Read the model definition and answer for the solid it produces. Units are mm, in the model's axes. Give positions to 0.01 mm unless a question says otherwise; leave off trailing zeros. Write each loop counter-clockwise with the first axis right and the second up, starting at its lowest first coordinate (ties: lowest second). Pieces come first, ordered by that corner, then holes. Notation, with made-up numbers: (7, 81) - (41, 81) arc R27 cw to (41, 108) - close; hole circle Ø6 at (1.5, -22). An arc over 180 degrees is marked (long way). Answer as a JSON object with one key per item and string values. Group by question number.
```python
from build123d import *

# Parameters (mm, degrees)
SKETCH1_R           = 17.5
BOSS_EXTRUDE1_DEPTH = 1.5
SKETCH2_R           = 7
SKETCH2_R_2         = 1.5
CUT_EXTRUDE1_DEPTH  = 1.5
CHAMFER1_SIZE       = 0.75
CHAMFER2_SIZE       = 0.25


with BuildPart() as part:
    # Sketch1 → Boss-Extrude1 (new body)
    with BuildSketch(Plane.XY):
        Circle(SKETCH1_R)
    extrude(amount=BOSS_EXTRUDE1_DEPTH)

    # Sketch2 → Cut-Extrude1 (cut)
    with BuildSketch(Plane.XY.offset(1.5)):
        with Locations((0, -3.5)):
            Circle(SKETCH2_R)
        with Locations((-8, 9.5)):
            Circle(SKETCH2_R_2)
        with Locations((8, 9.5)):
            Circle(SKETCH2_R_2)
    extrude(amount=-CUT_EXTRUDE1_DEPTH, mode=Mode.SUBTRACT)

    # Chamfer1
    chamfer1_edges = [part.edges().sort_by_distance(p)[0] for p in [
        (-9.5, 9.5, 1.5),
        (6.5, 9.5, 1.5),
    ]]
    chamfer(chamfer1_edges, length=CHAMFER1_SIZE)

    # Chamfer2
    chamfer2_edges = [part.edges().sort_by_distance(p)[0] for p in [
        (-17.5, 0, 0),
        (-17.5, 0, 1.5),
    ]]
    chamfer(chamfer2_edges, length=CHAMFER2_SIZE)


solid = part.part
```
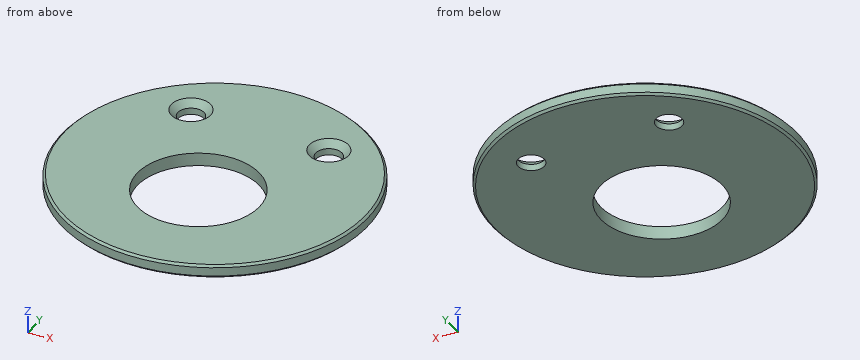
1) Find the intervals of material crossed by line 1 (Y direction, x = 0, z = 0.6); line 2 (X direction, y = 10, z = 0.15); line 3 (Y direction, x = 8, z = 0.35), in increasing order. Write a range as [from, to].
2) Find section C-C, the plane z = 0.5. Write down the section's boundary in (x, y).
3) A flat-ended cylindrical pin translates along its axis: pin 1 Ø11 at (x, y) = (0, -3.5) entering from +Z. Find the tip coordinate at first contact, or state that the pin passes through.
4) Find section B-B, the plane y = 0. Write down the section's boundary in (x, z), and give its area (3 significant figures).
5) Find section A-A, the plane x = 0. Write down the section's boundary in (y, z), and give its area (3 significant figures).
Values follow:
{
 "1": {"line 1": "y = [-17.5, -10.5], [3.5, 17.5]", "line 2": "x = [-14.24, -9.41], [-6.59, 6.59], [9.41, 14.24]", "line 3": "y = [-15.56, 8], [11, 15.56]"},
 "2": {"outline": "circle Ø35 at (0, 0); hole circle Ø3 at (-8, 9.5); hole circle Ø14 at (0, -3.5); hole circle Ø3 at (8, 9.5)"},
 "3": {"pin 1": "passes through"},
 "4": {"outline": "(-17.5, 0.25) - (-17.25, 0) - (-6.06, 0) - (-6.06, 1.5) - (-17.25, 1.5) - (-17.5, 1.25) - close; (6.06, 0) - (17.25, 0) - (17.5, 0.25) - (17.5, 1.25) - (17.25, 1.5) - (6.06, 1.5) - close", "area": "34.2 mm2"},
 "5": {"outline": "(-17.5, 0.25) - (-17.25, 0) - (-10.5, 0) - (-10.5, 1.5) - (-17.25, 1.5) - (-17.5, 1.25) - close; (3.5, 0) - (17.25, 0) - (17.5, 0.25) - (17.5, 1.25) - (17.25, 1.5) - (3.5, 1.5) - close", "area": "31.4 mm2"}
}
